CAD build for the part. Positions are in the model's coordinates, mm. Face numbers are marked on the shaded views. A direction names the side the tool comes from. Give positions to 0.01 mm unless a question says otherwise; leave off trailing zeros. Write each loop counter-clockwise with the first axis right and the second up, starting at its lowest first coordinate (ties: lowest second). Pieces come first, ordered by that corner, then holes. Notation, with made-up numbers: (-22.75, 17) - (-15.75, 17) arc R30 ccw to (-15.75, 52) - close; hole circle Ø9 at (17.25, 8.25). An arc over 180 degrees is marked (long way). Answer as a JSON object with one key per item and string values.
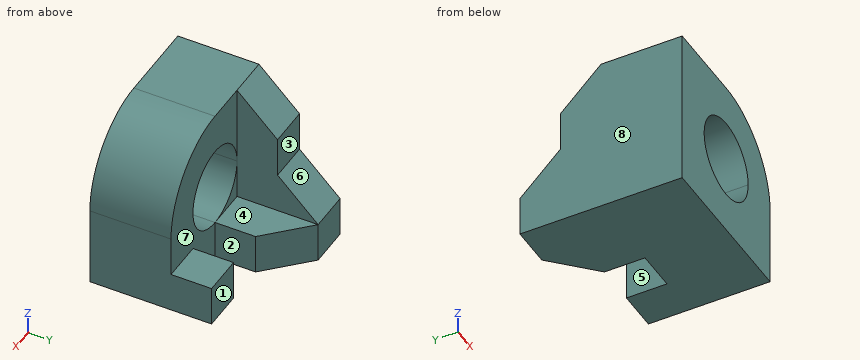
from build123d import *

# Parameters (mm, degrees)
SKETCH1_W               = 10
SKETCH1_H               = 10
BOSS_EXTRUDE1_DEPTH     = 20
SKETCH1_3_W             = 10
SKETCH1_3_H             = 10
BOSS_EXTRUDE2_DEPTH     = 30
SKETCH1_4_W             = 10
SKETCH1_4_H             = 10
BOSS_EXTRUDE3_DEPTH     = 40
CUT_EXTRUDE1_DEPTH      = 31
CUT_EXTRUDE1_DEPTH_BACK = 10
CUT_EXTRUDE2_DEPTH      = 31
CUT_EXTRUDE2_DEPTH_BACK = 10


with BuildPart() as part:
    # Sketch1 → Boss-Extrude1 (new body)
    with BuildSketch(Plane(origin=(0, 0, 0), x_dir=(1, 0, 0), z_dir=(0, 1, 0))):
        Polygon((10, 0), (0, 0), (0, -40), (10, -40), (10, -20), (10, -10), align=None)
        with BuildLine():
            Line((10, -20), (10, -40))
            Line((10, -40), (20, -40))
            ThreePointArc((20, -40), (34.142135624, -34.142135624), (40, -20))
            Line((40, -20), (40, -10))
            Line((40, -10), (30, -10))
            Line((30, -10), (30, 0))
            Line((30, 0), (20, 0))
            Line((20, 0), (20, -10))
            ThreePointArc((20, -10), (27.071067812, -12.928932188), (30, -20))
            ThreePointArc((30, -20), (20, -30), (10, -20))
        make_face()
        with Locations((15, -5)):
            Rectangle(SKETCH1_W, SKETCH1_H)
        with Locations((35, -5)):
            Rectangle(SKETCH1_W, SKETCH1_H)
        with BuildLine():
            Line((20, -10), (10, -10))
            Line((10, -10), (10, -20))
            ThreePointArc((10, -20), (12.928932188, -12.928932188), (20, -10))
        make_face()
    extrude(amount=BOSS_EXTRUDE1_DEPTH)

    # Sketch1<3> → Boss-Extrude2 (add)
    with BuildSketch(Plane(origin=(0, 0, 0), x_dir=(1, 0, 0), z_dir=(0, 1, 0))):
        with Locations((35, -5)):
            Rectangle(SKETCH1_3_W, SKETCH1_3_H)
    extrude(amount=BOSS_EXTRUDE2_DEPTH)

    # Sketch1<4> → Boss-Extrude3 (add)
    with BuildSketch(Plane(origin=(0, 0, 0), x_dir=(1, 0, 0), z_dir=(0, 1, 0))):
        with Locations((15, -5)):
            Rectangle(SKETCH1_4_W, SKETCH1_4_H)
        Polygon((10, 0), (0, 0), (0, -40), (10, -40), (10, -20), (10, -10), align=None)
    extrude(amount=BOSS_EXTRUDE3_DEPTH)

    # Sketch2 → Cut-Extrude1 (cut, two sides)
    with BuildSketch(Plane.XY.offset(10)) as cut_extrude1_sk:
        Polygon((20, 40), (10, 40), (20, 30), align=None)
    extrude(amount=CUT_EXTRUDE1_DEPTH, mode=Mode.SUBTRACT)
    extrude(cut_extrude1_sk.sketch, amount=-CUT_EXTRUDE1_DEPTH_BACK, mode=Mode.SUBTRACT)

    # Sketch3 → Cut-Extrude2 (cut, two sides)
    with BuildSketch(Plane(origin=(10, 0, 0), x_dir=(0, 0, -1), z_dir=(1, 0, 0))) as cut_extrude2_sk:
        Polygon((-117.781745931, -57.781745931), (-40, 20), (-30, 30), (-20, 30), (-10, 40), (67.781745931, 117.781745931), (-83.416065326, 277.591701412), (-268.979557187, 102.028209551), align=None)
    extrude(amount=CUT_EXTRUDE2_DEPTH, mode=Mode.SUBTRACT)
    extrude(cut_extrude2_sk.sketch, amount=-CUT_EXTRUDE2_DEPTH_BACK, mode=Mode.SUBTRACT)


solid = part.part
Item 1: Cut at A-A (z = 14). Give the cut face in (x, y).
Entries:
{"outline": "(0, 0) - (12, 0) - (12, 20) - (10, 20) - (10, 36) - (0, 36) - close; (28, 0) - (40, 0) - (40, 20) - (28, 20) - close"}
Item 2: Probe line 1 (X direction, y = 28, z = 8); line 2 (Z direction, x = 12.5, y = 20.5); line 3 (Y direction, x = 32, z = 7). List the from-to ranges inside material, lowest first. Write a range as from..to.
Entries:
{"line 1": "0..20, 30..40", "line 2": "0..10", "line 3": "0..30"}
Item 3: Cut at C-C (y = 17.5). Give the cut face in (x, z).
Entries:
{"outline": "(0, 0) - (40, 0) - (40, 20) arc R20 ccw to (20, 40) - (0, 40) - close; hole circle Ø20 at (20, 20)"}
Item 4: Which spindle directions (+Z, -Z, +X, -X, +Y, -Y) get a long thin tool onto all of the face, cutting with end or side? Do the marked faces 1, 2, 3 and 4. Say none if no direction does.
Entries:
{"face 1": "+Z, -Z, +X, +Y", "face 2": "+Z, -Z, +Y", "face 3": "+Z, +X, -X, +Y", "face 4": "+Z, +X, +Y"}
Item 5: Cut at B-B (x = 14). Give the cut face in (y, z), and give its area (3 significant figures).
Entries:
{"outline": "(0, 0) - (36, 0) - (36, 10) - (20, 10) - (20, 12) - (0, 12) - close; (0, 28) - (20, 28) - (20, 40) - (0, 40) - close", "area": "640 mm2"}
Item 6: Mould opens along X. For the marked faces 5, 6, 7 and 8 say: +X half, -X half, draft (parallel to the pull), parting line (faces both ways), or undercut.
Entries:
{"face 5": "undercut", "face 6": "draft", "face 7": "undercut", "face 8": "-X half"}
Item 7: Flat gauge pins, fed straight in: P1, Ø3, axis at x = 37.5, y = 25, coming from the +Z side; P2, Ø8, axis at x = 3, z = 26.5, coming from the +Y side; P3, Ø9, axis at x = 24.5, z = 29, coming from the +Y side; P4, Ø3, axis at x = 13, z = 16.5, coming from the +Y side. Where does each tip first touch, or does it go through?
Entries:
{"P1": "z = 10", "P2": "y = 30", "P3": "y = 20", "P4": "through"}
Item 8: Cut at D-D (y = 36.5). Give the cut face in (x, z), and give its area (3 significant figures).
Entries:
{"outline": "(0, 0) - (13.5, 0) - (13.5, 10) - (10, 10) - (10, 13.5) - (0, 13.5) - close", "area": "170 mm2"}
